Autodesk Inventor part; units mm, degrees
ref_plane "YZ Plane" through (0, 0, 0) normal (1, 0, 0) x (0, 1, 0)
ref_plane "XZ Plane" through (0, 0, 0) normal (0, 1, 0) x (-1, 0, 0)
ref_plane "XY Plane" through (0, 0, 0) normal (0, 0, 1) x (1, 0, 0)
sketch "Sketch1" plane through (0, 0, 0) normal (0, 0, 1) x (1, 0, 0)
  line L0 (0, 0) -> (4.0132, 0)
  line L1 (4.0132, 0) -> (4.0132, 6.477)
  line L2 (4.0132, 6.477) -> (0, 6.477)
  line L3 (0, 6.477) -> (0, 0)
  line L4 (0, 6.477) -> (4.826, 6.477)
  line L5 (4.826, 6.477) -> (4.826, 9.525)
  line L6 (4.826, 9.525) -> (0, 9.525)
  line L7 (0, 9.525) -> (0, 6.477)
  line L8 (0, 9.525) -> (3.3655, 9.525)
  line L9 (3.3655, 9.525) -> (3.3655, 17.399)
  line L10 (3.3655, 17.399) -> (0, 17.399)
  line L11 (0, 17.399) -> (0, 9.525)
  dimension "d0" = 4.0132
  dimension "d1" = 6.477
  dimension "d2" = 4.826
  dimension "d3" = 3.048
  dimension "d4" = 3.3655
  dimension "d5" = 7.874
revolve "Revolution1" add sketch "Sketch1" angle 360 about axis through (0, 17.399, 0) along (0, -1, 0)
thread "Thread1"
sketch "Sketch2" plane through (0, 0, 0) normal (0, -1, 0) x (1, 0, 0)
  line L0 (1.9693, -2.286) -> (-1.8407, -2.286)
  line L1 (-1.8407, -2.286) -> (-1.8407, -2.4989)
  line L2 (-1.8407, -2.4989) -> (1.9693, -2.4989)
  line L3 (1.9693, -2.4989) -> (1.9693, -2.286)
  line L4 (3.0926, 0) -> (-3.1405, 0)
  line L5 (1.9693, 2.286) -> (-1.8407, 2.286)
  line L6 (-1.8407, 2.286) -> (-1.8407, 2.4989)
  line L7 (-1.8407, 2.4989) -> (1.9693, 2.4989)
  line L8 (1.9693, 2.4989) -> (1.9693, 2.286)
  point P0 (0, 0)
  dimension "d9" = 3.81
  dimension "d10" = 2.286
extrude "Extrusion1" add sketch "Sketch2" along normal blind 7.874
properties part number "PushSwitchBody" material "Stainless Steel"
Verification items for the finished model (mm, model axes). A direction names the side the tool comes from. Give positions to 0.01 mm unless a question says otherwise; leave off trailing zeros. Write each loop counter-clockwise with the first axis right and the second up, starting at its lowest first coordinate (ties: lowest second). Pieces come first, ordered by that corner, then holes. Notation, with made-up numbers: M -35.5,33 L 7.5,33 A20 ccw 7.5,59 Z; hole C 57,-15.75 d2. An arc over 180 degrees is marked long. One line per question, with ' | ' between items.
1) Mould release check, pull along Z, two halves, no side actions. Record for faces 1 (the flat face through (0, -4, -2.499)), 2 (the flat face through (0, 0, 0)), 3 (the flat face through (0, -4, -2.286)), 4 (the flat face through (0, 17.399, 0)): released by +Z, released by -Z, zero draft, split by the parting line, or undercut.
Result:
face 1: released by -Z | face 2: undercut | face 3: undercut | face 4: zero draft
2) Section check D-D on y = 14. Enter the section's corners in (x, z), plus the area to 3 significant figures.
Result:
outline: C 0,0 d6.73 | area: 35.6 mm2
3) Thickness scan on line 1 along Z through (x, y) = (-0.25, -2.5); line 2 along Y through (x, z) = (-0.75, 3); line 3 along Z through (x, y) = (-2.75, 13.5). Record the ranges inside material, lowest first. Write a range as [from, to].
Result:
line 1: z = [-2.5, -2.29], [2.29, 2.5] | line 2: y = [0, 17.4] | line 3: z = [-1.94, 1.94]
4) Section check A-A on y = -5.5. Enter the section's corners in (x, z).
Result:
outline: M -1.84,-2.5 L 1.97,-2.5 L 1.97,-2.29 L -1.84,-2.29 Z; M -1.84,2.29 L 1.97,2.29 L 1.97,2.5 L -1.84,2.5 Z
5) Set-up check for faces 5 (the flat face through (0, -4, 2.286)), 6 (the flat face through (0, -4, 2.499)), 7 (the cylindrical face through (-2.67, 13.52, 2.05)): record each of +Z, -Z, +X, -X, +Y, -Y from which the full face is reachable in a straight line by a thin tool's end or side.
Result:
face 5: +X, -X, -Y | face 6: +Z, +X, -X, -Y | face 7: +Y
6) Section check B-B on z = 0. Enter the section's corners in (x, y) (1 decimal).
Result:
outline: M -4.8,6.5 L -4,6.5 L -4,0 L 4,0 L 4,6.5 L 4.8,6.5 L 4.8,9.5 L 3.4,9.5 L 3.4,17.4 L -3.4,17.4 L -3.4,9.5 L -4.8,9.5 Z
7) Gauge pin test, flat ends, axial feed: pin 1 Ø1.1 at (x, y) = (0, -5.5) entering from +Z; pin 2 Ø3 at (x, z) = (3.5, -0.5) entering from -Y; pin 3 Ø2 at (x, y) = (-3.5, 3) entering from +Z. Record the tip position at first contact, or that the pin passes through.
Result:
pin 1: stops at z = 2.5 | pin 2: stops at y = 0 | pin 3: stops at z = 3.14
